```python
from build123d import *

# Parameters (mm, degrees)
SKETCH1_W           = 30
SKETCH1_H           = 52
BOSS_EXTRUDE1_DEPTH = 25
SKETCH2_R           = 9
BOSS_EXTRUDE2_DEPTH = 3
CHAMFER1_SIZE       = 3
SKETCH3_R           = 5
BOSS_EXTRUDE3_DEPTH = 1
SKETCH4_R           = 1.75
CUT_EXTRUDE1_DEPTH  = 67.970142601


with BuildPart() as part:
    # Sketch1 → Boss-Extrude1 (new body)
    with BuildSketch(Plane(origin=(0, 0, 0), x_dir=(1, 0, 0), z_dir=(0, 1, 0))):
        with Locations((15, 26)):
            Rectangle(SKETCH1_W, SKETCH1_H)
    extrude(amount=BOSS_EXTRUDE1_DEPTH)

    # Sketch2 → Boss-Extrude2 (add)
    with BuildSketch(Plane(origin=(30, 0, 0), x_dir=(0, 0, -1), z_dir=(1, 0, 0))):
        with Locations((13.5, 13.021886364)):
            Circle(SKETCH2_R)
        with Locations(Location((38.5, 13.021886364, 0), (0, 0, 180))):
            Circle(SKETCH2_R)
    extrude(amount=BOSS_EXTRUDE2_DEPTH)

    # Chamfer1
    chamfer1_edges = [part.edges().sort_by_distance(p)[0] for p in [
        (33, 13.021886364, -4.5),
        (33, 13.021886364, -47.5),
    ]]
    chamfer(chamfer1_edges, length=CHAMFER1_SIZE - 0.0001)  # a hair under: the kernel refuses the full size

    # Sketch3 → Boss-Extrude3 (add)
    with BuildSketch(Plane(origin=(33, 0, 0), x_dir=(0, 0, -1), z_dir=(1, 0, 0))):
        with Locations((38.5, 13.021886364)):
            Circle(SKETCH3_R)
        with Locations((13.5, 13.021886364)):
            Circle(SKETCH3_R)
    extrude(amount=BOSS_EXTRUDE3_DEPTH)

    # Sketch4 → Cut-Extrude1 (cut, through all)
    with BuildSketch(Plane.XZ):
        with Locations(Location((15, -26, 0), (0, 0, 270))):
            Circle(SKETCH4_R)
    extrude(amount=-CUT_EXTRUDE1_DEPTH, mode=Mode.SUBTRACT)


solid = part.part
```
Model file for the job. Use its own axes, mm. A direction names the side the tool comes from. Give positions to 0.01 mm unless a question says otherwise; leave off trailing zeros. Write each loop counter-clockwise with the first axis right and the second up, starting at its lowest first coordinate (ties: lowest second). Pieces come first, ordered by that corner, then holes. Notation, with made-up numbers: M 41,44.25 L 71,44.25 A26 cw 71,58.25 Z; hole C 86,-5 d10. An arc over 180 degrees is marked long. Use a Markdown table: item, result.
1) Tool access for faces 1 (the cylindrical face through (33.49, 14.52, -18.27)), 2 (the cylindrical face through (16.18, 12.32, -24.71)): list every direction of +Z, -Z, +X, -X, +Y, -Y with a clear straight run to the whole face (end or side of a thin tool).
Responses:
| item | result |
|---|---|
| face 1 | +X |
| face 2 | +Y, -Y |
2) Drill centre lines: line 1 (X direction, y = 19.75, z = -26); line 2 (X direction, y = 19, z = -6.5); line 3 (X direction, y = 18.5, z = -39.5). Where is each one in solid material? Low to high. Write a range as from..to.
Responses:
| item | result |
|---|---|
| line 1 | x = 0..13.25, 16.75..30 |
| line 2 | x = 0..30 |
| line 3 | x = 0..33 |
3) Pin check, flat tip, straight feed: pin 1 (2 mm diameter, centred on x = 18, z = -42.5, fed in from -Y). Stop position of the tip, or through.
Responses:
| item | result |
|---|---|
| pin 1 | stops at y = 0 |
4) Cut at A-A (x = 15). List the corners of the cut face in (y, z).
Responses:
| item | result |
|---|---|
| outline | M 0,-52 L 25,-52 L 25,-27.75 L 0,-27.75 Z; M 0,-24.25 L 25,-24.25 L 25,0 L 0,0 Z |
5) Pull direction Z, two halves, no side cores. Call faces 3 (the flat face through (34, 13, -38)), 4 (the conical face through (32.854, 11.176, -32.638)), 5 (the flat face through (15, 12, -52)), 6 (the flat face through (33, 18, -12)): +Z half, -Z half, draft (parallel to the pull), parting line (faces both ways), or undercut.
Responses:
| item | result |
|---|---|
| face 3 | draft |
| face 4 | undercut |
| face 5 | -Z half |
| face 6 | undercut |
